from build123d import *

# Parameters (mm, degrees)
SKETCH_1_W          = 50
SKETCH_1_H          = 50
SKETCH_1_R          = 21.05
EXTRUDE_1_DEPTH     = 15
SKETCH_2_W          = 50
SKETCH_2_H          = 30
SKETCH_2_R          = 1.6
EXTRUDE_2_DEPTH     = 15
FILLET_1_R          = 3
SKETCH_3_R          = 1.75
CUT_EXTRUDE_1_DEPTH = 63.24949799
SKETCH_4_R          = 1.6
CUT_EXTRUDE_2_DEPTH = 63.24949799
FILLET_2_R          = 2
FILLET_3_R          = 5
SKETCH_5_W          = 22
SKETCH_5_H          = 10
CUT_EXTRUDE_3_DEPTH = 50.497474683
FILLET_4_R          = 1


with BuildPart() as part:
    # 草图1 → 凸台-拉伸1 (new body)
    with BuildSketch(Plane(origin=(0, 0, 0), x_dir=(1, 0, 0), z_dir=(0, 1, 0))):
        Rectangle(SKETCH_1_W, SKETCH_1_H)
        with Locations(Location((0, 0, 0), (0, 0, 270))):
            Circle(SKETCH_1_R, mode=Mode.SUBTRACT)
    extrude(amount=EXTRUDE_1_DEPTH)

    # 草图2 → 凸台-拉伸2 (add)
    with BuildSketch(Plane(origin=(0, 15, 0), x_dir=(1, 0, 0), z_dir=(0, 1, 0))):
        with Locations((0, -40)):
            Rectangle(SKETCH_2_W, SKETCH_2_H)
        with Locations(Location((-15, -47.5, 0), (0, 0, 270))):
            Circle(SKETCH_2_R, mode=Mode.SUBTRACT)
        with Locations(Location((15, -47.5, 0), (0, 0, 270))):
            Circle(SKETCH_2_R, mode=Mode.SUBTRACT)
    extrude(amount=-EXTRUDE_2_DEPTH)

    # 圆角1
    fillet_1_edges = [part.edges().sort_by_distance(p)[0] for p in [
        (25, 7.5, 55),
        (-25, 7.5, 55),
        (-25, 7.5, -25),
        (25, 7.5, -25),
    ]]
    fillet(fillet_1_edges, radius=FILLET_1_R)

    # 草图3 → 切除-拉伸1 (cut, through all)
    with BuildSketch(Plane(origin=(0, 15, 0), x_dir=(1, 0, 0), z_dir=(0, 1, 0))):
        with Locations(Location((-15, -30, 0), (0, 0, 270))):
            Circle(SKETCH_3_R)
        with Locations(Location((15, -30, 0), (0, 0, 270))):
            Circle(SKETCH_3_R)
    extrude(amount=-CUT_EXTRUDE_1_DEPTH, mode=Mode.SUBTRACT)

    # 草图4 → 切除-拉伸2 (cut, through all)
    # profile 1 of 6: a face of its own
    with BuildSketch(Plane(origin=(0, 15, 0), x_dir=(1, 0, 0), z_dir=(0, 1, 0))):
        with BuildLine():
            Line((25, -40), (-25, -40))
            Line((-25, -40), (-25, -52))
            ThreePointArc((-25, -52), (-24.121320344, -54.121320344), (-22, -55))
            Line((-22, -55), (22, -55))
            ThreePointArc((22, -55), (24.121320344, -54.121320344), (25, -52))
            Line((25, -52), (25, -40))
        make_face()
        with Locations((-15, -47.5)):
            Circle(SKETCH_4_R, mode=Mode.SUBTRACT)
        with Locations((15, -47.5)):
            Circle(SKETCH_4_R, mode=Mode.SUBTRACT)
    # profile 2 of 6: a face of its own
    with BuildSketch(Plane(origin=(0, 15, 0), x_dir=(1, 0, 0), z_dir=(0, 1, 0))):
        with BuildLine():
            Line((-25, 22), (-25, -12))
            Line((-25, -12), (-20.784609691, -12))
            ThreePointArc((-20.784609691, -12), (-6.211657082, 23.182219831), (24, 0))
            ThreePointArc((24, 0), (23.182219831, -6.211657082), (20.784609691, -12))
            Line((20.784609691, -12), (25, -12))
            Line((25, -12), (25, 22))
            ThreePointArc((25, 22), (24.121320344, 24.121320344), (22, 25))
            Line((22, 25), (-22, 25))
            ThreePointArc((-22, 25), (-24.121320344, 24.121320344), (-25, 22))
        make_face()
    # profile 3 of 6: a face of its own
    with BuildSketch(Plane(origin=(0, 15, 0), x_dir=(1, 0, 0), z_dir=(0, 1, 0))):
        with BuildLine():
            ThreePointArc((24, 0), (-6.211657082, 23.182219831), (-20.784609691, -12))
            Line((-20.784609691, -12), (-17.294580076, -12))
            ThreePointArc((-17.294580076, -12), (-6.286954326, 20.089218633), (21.05, 0))
            ThreePointArc((21.05, 0), (20.089218633, -6.286954326), (17.294580076, -12))
            Line((17.294580076, -12), (20.784609691, -12))
            ThreePointArc((20.784609691, -12), (23.182219831, -6.211657082), (24, 0))
        make_face()
    # profile 4 of 6: a face of its own
    with BuildSketch(Plane(origin=(0, 15, 0), x_dir=(1, 0, 0), z_dir=(0, 1, 0))):
        with BuildLine():
            Line((-17.294580076, -12), (-20.784609691, -12))
            ThreePointArc((-20.784609691, -12), (0, -24), (20.784609691, -12))
            Line((20.784609691, -12), (17.294580076, -12))
            ThreePointArc((17.294580076, -12), (0, -21.05), (-17.294580076, -12))
        make_face()
    # profile 5 of 6: a face of its own
    with BuildSketch(Plane(origin=(0, 15, 0), x_dir=(1, 0, 0), z_dir=(0, 1, 0))):
        with BuildLine():
            ThreePointArc((24, 0), (-6.211657082, 23.182219831), (-20.784609691, -12))
            Line((-20.784609691, -12), (-17.294580076, -12))
            ThreePointArc((-17.294580076, -12), (-6.286954326, 20.089218633), (21.05, 0))
            ThreePointArc((21.05, 0), (20.089218633, -6.286954326), (17.294580076, -12))
            Line((17.294580076, -12), (20.784609691, -12))
            ThreePointArc((20.784609691, -12), (23.182219831, -6.211657082), (24, 0))
        make_face()
    # profile 6 of 6: a face of its own
    with BuildSketch(Plane(origin=(0, 15, 0), x_dir=(1, 0, 0), z_dir=(0, 1, 0))):
        with BuildLine():
            Line((-17.294580076, -12), (-20.784609691, -12))
            ThreePointArc((-20.784609691, -12), (0, -24), (20.784609691, -12))
            Line((20.784609691, -12), (17.294580076, -12))
            ThreePointArc((17.294580076, -12), (0, -21.05), (-17.294580076, -12))
        make_face()
    extrude(amount=-CUT_EXTRUDE_2_DEPTH, mode=Mode.SUBTRACT)

    # 圆角2
    fillet_2_edges = [part.edges().sort_by_distance(p)[0] for p in [
        (20.784609691, 7.5, 12),
        (-20.784609691, 7.5, 12),
        (-25, 7.5, 12),
        (25, 7.5, 12),
    ]]
    fillet(fillet_2_edges, radius=FILLET_2_R)

    # 圆角3
    fillet_3_edges = [part.edges().sort_by_distance(p)[0] for p in [
        (-25, 7.5, 40),
        (25, 7.5, 40),
    ]]
    fillet(fillet_3_edges, radius=FILLET_3_R)

    # 草图5 → 切除-拉伸3 (cut, through all)
    with BuildSketch(Plane(origin=(0, 15, 0), x_dir=(1, 0, 0), z_dir=(0, 1, 0))):
        with Locations((0, -32.5)):
            Rectangle(SKETCH_5_W, SKETCH_5_H)
    extrude(amount=-CUT_EXTRUDE_3_DEPTH, mode=Mode.SUBTRACT)

    # 圆角4
    fillet_4_edges = [part.edges().sort_by_distance(p)[0] for p in [
        (11, 0, 32.5),
        (11, 7.5, 27.5),
        (0, 0, 37.5),
        (11, 7.5, 37.5),
        (-11, 0, 32.5),
        (-11, 7.5, 37.5),
        (0, 0, 27.5),
        (-11, 7.5, 27.5),
        (11, 15, 32.5),
        (0, 15, 27.5),
        (-11, 15, 32.5),
        (0, 15, 37.5),
    ]]
    fillet(fillet_4_edges, radius=FILLET_4_R)


solid = part.part
The listing builds one solid part. Answer for the finished solid, in the listing's coordinates (mm). A direction names the side the tool comes from. Coordinates: 2 decimals unless noted, no trailing zeros. Loops run counter-clockwise (first coordinate to the right, second up) from the corner with the lowest first, then second, coordinate; pieces in that order, holes last. Notation, with made-up numbers: M 11.5,-25 L 62.5,-25 A23 cw 62.5,1 Z; hole C 81.25,49 d8. An arc over 180 degrees is marked long. Answer in a Markdown table with one row per item.
1) Determine the mould class of faces 1 (the cylindrical face through (10.715, 7.409, 27.801)), 2 (the cylindrical face through (-24.43, 7.4, 12.6)), 3 (the flat face through (-25, 8, 25)) for opening direction Z: released by +Z, released by -Z, zero draft, split by the parting line, or undercut.
Answers below:
| item | result |
|---|---|
| face 1 | undercut |
| face 2 | released by -Z |
| face 3 | zero draft |
2) Find section A-A (z = 30). Determine the outline of the cut face in (x, y), then the cut area to 3 significant figures.
Answers below:
| item | result |
|---|---|
| outline | M -25,0 L -16.75,0 L -16.75,15 L -25,15 Z; M -13.25,0 L -12,0 A1 ccw -11,1 L -11,14 A1 ccw -12,15 L -13.25,15 Z; M 11,1 A1 ccw 12,0 L 13.25,0 L 13.25,15 L 12,15 A1 ccw 11,14 Z; M 16.75,0 L 25,0 L 25,15 L 16.75,15 Z |
| area | 314 mm^2 |
3) Find section D-D (x = -15). Determine the outline of the cut face in (y, z) (3 decimals), then the cut area to 3 significant figures.
Answers below:
| item | result |
|---|---|
| outline | M 0,18.735 L 15,18.735 L 15,28.25 L 0,28.25 Z; M 0,31.75 L 15,31.75 L 15,40 L 0,40 Z |
| area | 266 mm^2 |
4) Find section B-B (z = 34). Determine the outline of the cut face in (x, y).
Answers below:
| item | result |
|---|---|
| outline | M -25,0 L -12,0 A1 ccw -11,1 L -11,14 A1 ccw -12,15 L -25,15 Z; M 11,1 A1 ccw 12,0 L 25,0 L 25,15 L 12,15 A1 ccw 11,14 Z |
5) Given pin 1 (6 mm diameter, centred on x = 0, y = 8, fed in from -Z); pin 2 (4 mm diameter, centred on x = -15, z = 30, fed in from -Y); pin 3 (3 mm diameter, centred on x = 15, z = 30, fed in from -Y); pin 4 (8 mm diameter, centred on x = 4, y = 10, fed in from -Z), each flat-ended and moving along its own axis, determine where each tip first touches the part or whether it passes through.
Answers below:
| item | result |
|---|---|
| pin 1 | z = 23.81 |
| pin 2 | y = 0 |
| pin 3 | through |
| pin 4 | z = 22.63 |
6) Find section C-C (y = 6). Determine the outline of the cut face in (x, z), then the cut area to 3 significant figures.
Answers below:
| item | result |
|---|---|
| outline | M -25,14 A2 ccw -23,12 L -21.91,12 A2 ccw -20.22,12.92 A24 cw 20.22,12.92 A2 ccw 21.91,12 L 23,12 A2 ccw 25,14 L 25,35 A5 ccw 20,40 L -20,40 A5 ccw -25,35 Z; hole C -15,30 d3.5; hole M -11,28.5 A1 ccw -10,27.5 L 10,27.5 A1 ccw 11,28.5 L 11,36.5 A1 ccw 10,37.5 L -10,37.5 A1 ccw -11,36.5 Z; hole C 15,30 d3.5 |
| area | 795 mm^2 |
7) Which of the six approach directions +Z, -Z, +X, -X, +Y, -Y give full straight-line access (tool end or side, diameter ignored) to faces 4 (the flat face through (0, 8, 27.5)), 5 (the cylindrical face through (11.301, 0.285, 32.444)), 6 (the cylindrical face through (0.14, 14.715, 27.199))?
Answers below:
| item | result |
|---|---|
| face 4 | +Y, -Y |
| face 5 | -Y |
| face 6 | +Y |
8) Find the intervals of material crossed by probe 1 along X at (y, z) = (10.5, 30); probe 2 along Z at (x, y) = (0, 4); probe 3 along X at (y, z) = (11.25, 37), in increasing order.
Answers below:
| item | result |
|---|---|
| probe 1 | -25 to -16.75, -13.25 to -11, 11 to 13.25, 16.75 to 25 |
| probe 2 | 24 to 27.5, 37.5 to 40 |
| probe 3 | -24.58 to -10.87, 10.87 to 24.58 |
